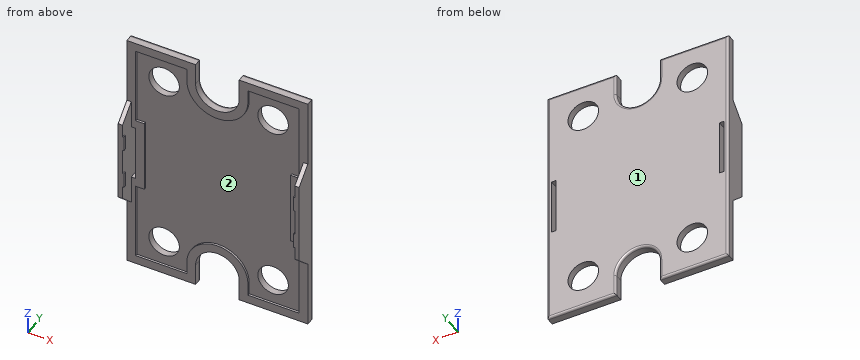
from build123d import *

# Parameters (mm, degrees)
SKETCH1_W           = 41.5
SKETCH1_H           = 57
BOSS_EXTRUDE1_DEPTH = 2
CUT_EXTRUDE1_DEPTH  = 3
SKETCH3_R           = 3.5
CUT_EXTRUDE2_DEPTH  = 3
SKETCH4_W           = 2
SKETCH4_H           = 13
CUT_EXTRUDE3_DEPTH  = 3
CUT_EXTRUDE4_DEPTH  = 0.5
BOSS_EXTRUDE2_DEPTH = 1
SKETCH7_W           = 3.5
SKETCH7_H           = 0.6
BOSS_EXTRUDE3_DEPTH = 0.3
FILLET1_R           = 0.5


with BuildPart() as part:
    # Sketch1 → Boss-Extrude1 (new body)
    with BuildSketch(Plane(origin=(0, 0, 0), x_dir=(1, 0, 0), z_dir=(0, 1, 0))):
        Rectangle(SKETCH1_W, SKETCH1_H)
    extrude(amount=BOSS_EXTRUDE1_DEPTH)

    # Sketch2 → Cut-Extrude1 (cut, through all)
    with BuildSketch(Plane(origin=(0, 2, 0), x_dir=(1, 0, 0), z_dir=(0, 1, 0))):
        with BuildLine():
            Line((-5, -23.5), (-5, -28.5))
            Line((-5, -28.5), (5, -28.5))
            Line((5, -28.5), (5, -23.5))
            ThreePointArc((5, -23.5), (0, -18.5), (-5, -23.5))
        make_face()
    cut_extrude1 = extrude(amount=-CUT_EXTRUDE1_DEPTH, mode=Mode.SUBTRACT)

    # Sketch3 → Cut-Extrude2 (cut, through all)
    with BuildSketch(Plane(origin=(0, 2, 0), x_dir=(1, 0, 0), z_dir=(0, 1, 0))):
        with Locations((-12.5, -20.75)):
            Circle(SKETCH3_R)
        with Locations((12.5, -20.75)):
            Circle(SKETCH3_R)
    cut_extrude2 = extrude(amount=-CUT_EXTRUDE2_DEPTH, mode=Mode.SUBTRACT)

    # Mirror1: Cut-Extrude1, Cut-Extrude2 across plane
    add(cut_extrude1.mirror(Plane.XY), mode=Mode.SUBTRACT)
    add(cut_extrude2.mirror(Plane.XY), mode=Mode.SUBTRACT)

    # Sketch4 → Cut-Extrude3 (cut, through all)
    with BuildSketch(Plane(origin=(0, 2, 0), x_dir=(1, 0, 0), z_dir=(0, 1, 0))):
        with Locations((-19.75, 0)):
            Rectangle(SKETCH4_W, SKETCH4_H)
        with Locations((19.75, 0)):
            Rectangle(SKETCH4_W, SKETCH4_H)
    extrude(amount=-CUT_EXTRUDE3_DEPTH, mode=Mode.SUBTRACT)

    # Sketch5 → Cut-Extrude4 (cut)
    with BuildSketch(Plane(origin=(0, 0, 0), x_dir=(1, 0, 0), z_dir=(0, 1, 0))):
        with BuildLine():
            Line((-18.75, 26.5), (-18.75, 8.5))
            Line((-18.75, 8.5), (-16.75, 8.5))
            Line((-16.75, 8.5), (-16.75, -8.5))
            Line((-16.75, -8.5), (-18.75, -8.5))
            Line((-18.75, -8.5), (-18.75, -26.5))
            Line((-18.75, -26.5), (-7, -26.5))
            Line((-7, -26.5), (-7, -23.5))
            ThreePointArc((-7, -23.5), (0, -16.5), (7, -23.5))
            Line((7, -23.5), (7, -26.5))
            Line((7, -26.5), (18.75, -26.5))
            Line((18.75, -26.5), (18.75, -8.5))
            Line((18.75, -8.5), (16.75, -8.5))
            Line((16.75, -8.5), (16.75, 8.5))
            Line((16.75, 8.5), (18.75, 8.5))
            Line((18.75, 8.5), (18.75, 26.5))
            Line((18.75, 26.5), (7, 26.5))
            Line((7, 26.5), (7, 23.5))
            ThreePointArc((7, 23.5), (0, 16.5), (-7, 23.5))
            Line((-7, 23.5), (-7, 26.5))
            Line((-7, 26.5), (-18.75, 26.5))
        make_face()
    extrude(amount=CUT_EXTRUDE4_DEPTH, mode=Mode.SUBTRACT)

    # Sketch6 → Boss-Extrude2 (add)
    with BuildSketch(Plane.ZY.offset(20.75)):
        Polygon((-13, 2), (13, 2), (13, 0), (9.5, -3.6), (-9.5, -3.6), (-13, 0), align=None)
    boss_extrude2 = extrude(amount=-BOSS_EXTRUDE2_DEPTH)

    # Sketch7 → Boss-Extrude3 (add)
    with BuildSketch(Plane(origin=(-19.75, 0, 0), x_dir=(0, 0, -1), z_dir=(1, 0, 0))):
        with Locations((-4.75, -3.3)):
            Rectangle(SKETCH7_W, SKETCH7_H)
        with Locations((4.75, -3.3)):
            Rectangle(SKETCH7_W, SKETCH7_H)
    boss_extrude3 = extrude(amount=BOSS_EXTRUDE3_DEPTH)

    # Mirror2: Boss-Extrude2, Boss-Extrude3 across plane
    add(boss_extrude2.mirror(Plane(origin=(0, 0, 0), x_dir=(0, 0, 1), z_dir=(1, 0, 0))))
    add(boss_extrude3.mirror(Plane(origin=(0, 0, 0), x_dir=(0, 0, 1), z_dir=(1, 0, 0))))

    # Fillet1
    fillet1_edges = [part.edges().sort_by_distance(p)[0] for p in [
        (-20.75, 2, 0),
        (-12.875, 2, 28.5),
        (12.875, 2, 28.5),
        (5, 2, 26),
        (0, 2, 18.5),
        (-5, 2, 26),
        (20.75, 2, 0),
        (-12.875, 2, -28.5),
        (5, 2, -26),
        (0, 2, -18.5),
        (-5, 2, -26),
        (12.875, 2, -28.5),
    ]]
    fillet(fillet1_edges, radius=FILLET1_R)


solid = part.part
Input: part model. Units: mm. Frame: model coordinates. Face numbers are marked on the shaded views. Coordinates: 2 decimals unless noted, no trailing zeros. Order: outer loops, then holes, each group sorted by start corner. A loop starts at its lowest first (then second) coordinate and runs counter-clockwise, first axis right, second up.
1. Cut plane A-A, the plane x = -12.5. Return loops of the section in (y, z).
Checked values:
outline: (0, -28.5) - (1.5, -28.5) arc R0.5 ccw to (2, -28) - (2, -24.25) - (0.5, -24.25) - (0.5, -26.5) - (0, -26.5) - close; (0, 26.5) - (0.5, 26.5) - (0.5, 24.25) - (2, 24.25) - (2, 28) arc R0.5 ccw to (1.5, 28.5) - (0, 28.5) - close; (0.5, -17.25) - (2, -17.25) - (2, 17.25) - (0.5, 17.25) - close
2. Cut plane C-C, the plane z = -14.5. Return loops of the section in (x, y), plus the area to 3 significant figures.
Checked values:
outline: (-20.75, 0) - (-18.75, 0) - (-18.75, 0.5) - (18.75, 0.5) - (18.75, 0) - (20.75, 0) - (20.75, 1.5) arc R0.5 ccw to (20.25, 2) - (-20.25, 2) arc R0.5 ccw to (-20.75, 1.5) - close
area: 64.1 mm2
3. Contact query for flat-ended pins moving along their axis: P1, Ø1.5, axis at x = -3.5, z = -7, coming from the -Y side; P2, Ø4, axis at x = 12.5, z = -20.75, coming from the -Y side. Output: stop coordinate, or through.
Checked values:
P1: stops at y = 0.5
P2: passes through
4. Cut plane B-B, the plane y = -0.65. Return loops of the section in (x, z).
Checked values:
outline: (-20.75, -12.37) - (-19.75, -12.37) - (-19.75, 12.37) - (-20.75, 12.37) - close; (19.75, -12.37) - (20.75, -12.37) - (20.75, 12.37) - (19.75, 12.37) - close
5. Ray query, line 1 along Z through (x, y) = (-12.5, 1.15); line 2 along X through (y, z) = (0.4, 24.5); line 3 along X through (y, z) = (-0.05, 11). Return the intervals inside material, ascending.
Checked values:
line 1: z = -28.5 to -24.25, -17.25 to 17.25, 24.25 to 28.5
line 2: x = -20.75 to -18.75, -7 to -5, 5 to 7, 18.75 to 20.75
line 3: x = -20.75 to -19.75, 19.75 to 20.75
6. Cut plane D-D, the plane z = -20.75. Count the separate pieces of the cut face and the enclosed holes in it, plus the area to 3 significant figures.
Checked values:
separate pieces: 4
enclosed holes: 0
area: 32.7 mm2
7. Draft query along X for the marked faces 1 and 2. Return one class per face: +X half, -X half, draft (parallel to the pull), parting line (faces both ways), or undercut.
Checked values:
face 1: draft
face 2: undercut
